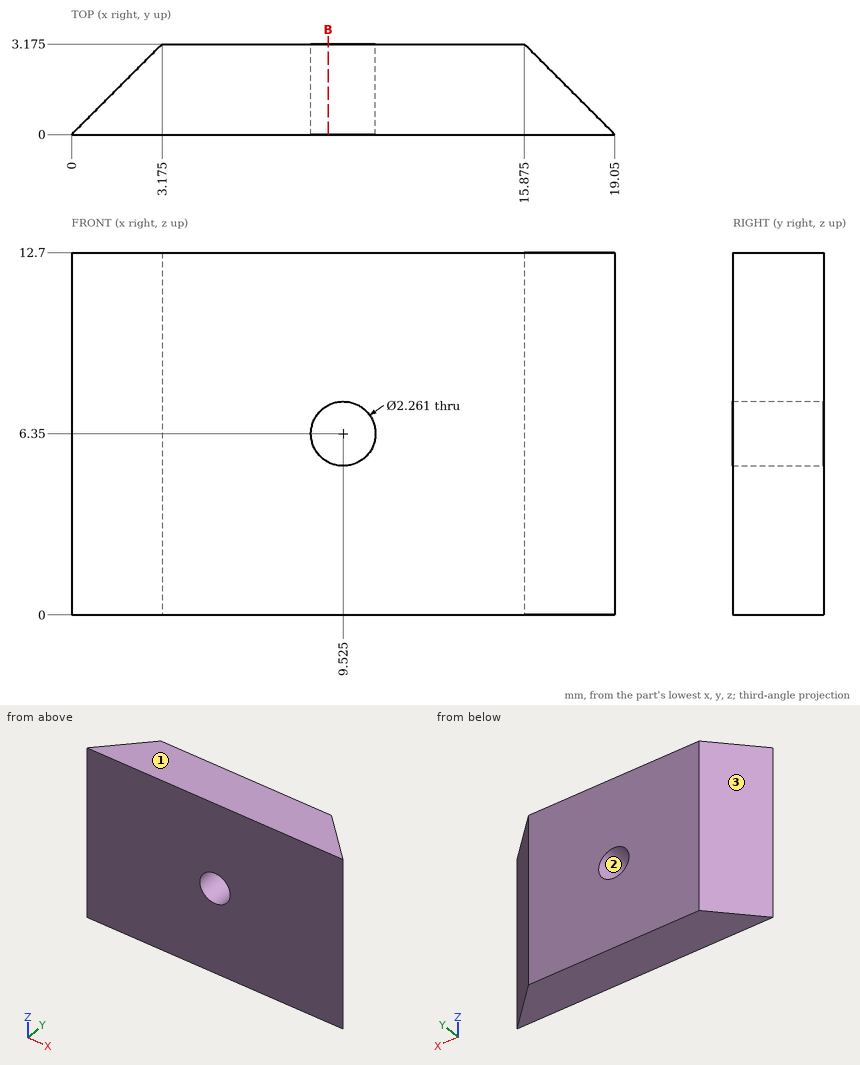
Print and shaded views of the part. All mm, measured from the part's lowest x, y and z. Coordinates: 2 decimals unless noted, no trailing zeros. Order: outer loops, then holes, each group sorted by start corner. A loop starts at its lowest first (then second) coordinate and runs counter-clockwise, first axis right, second up.
(1) Probe L1, parallel to Z at x = 8.5, y = 2.45 (1 decimal); L2, parallel to Z at x = 10, y = 1.95 (1 decimal); L3, parallel to X at y = 2.3, z = 7. List the from-to ranges inside material, lowest first.
Check sheet entries:
L1: z = 0 to 5.9, 6.8 to 12.7
L2: z = 0 to 5.3, 7.4 to 12.7
L3: x = 2.3 to 8.6, 10.45 to 16.75
(2) Pin check, flat tips, straight feed: pin 1 Ø1.4 at (x, z) = (9.525, 6.35) entering from +Y; pin 2 Ø1.5 at (y, z) = (2.5, 8.5) entering from -X. Stop position of each tip, or through.
Check sheet entries:
pin 1: passes through
pin 2: stops at x = 1.75
(3) Slice it at B-B, the plane x = 9. Write the cut outline in (y, z) (1 decimal).
Check sheet entries:
outline: (0, 0) - (3.2, 0) - (3.2, 5.3) - (0, 5.3) - close; (0, 7.4) - (3.2, 7.4) - (3.2, 12.7) - (0, 12.7) - close
(4) Pull direction X, two halves, no side cores. Call the marked faces 1, 2 and 3: pulls with the +X half, pulls with the -X half, needs draft (parallel to the pull), parting line crosses it, or undercut.
Check sheet entries:
face 1: needs draft
face 2: undercut
face 3: pulls with the -X half
